The listing builds one solid part. Answer for the finished solid, in the listing's coordinates (mm). A direction names the side the tool comes from. Round coordinates to 2 decimals unless told otherwise and drop trailing zeros. Write each loop counter-clockwise with the first axis right and the second up, starting at its lowest first coordinate (ties: lowest second). Pieces come first, ordered by that corner, then holes. Notation, with made-up numbers: (-27.75, 51) - (25.25, 51) arc R17 ccw to (25.25, 71) - close; hole circle Ø1 at (-15, -36.75). An arc over 180 degrees is marked (long way). Return JSON: item names as keys, results as strings. Group by question number.
from build123d import *

# Parameters (mm, degrees)
SKETCH_1_W          = 107
SKETCH_1_H          = 94
EXTRUDE_1_DEPTH     = 8.5
SKETCH_2_W          = 104
SKETCH_2_H          = 91
CUT_EXTRUDE_1_DEPTH = 6.5
SKETCH_3_W          = 100
SKETCH_3_H          = 5.5
CUT_EXTRUDE_2_DEPTH = 6
SKETCH_4_W          = 10
SKETCH_4_H          = 15
EXTRUDE_2_DEPTH     = 2
FILLET_1_R          = 2
SKETCH_5_R          = 1.5
CUT_EXTRUDE_3_DEPTH = 3


with BuildPart() as part:
    # 草图1 → 凸台-拉伸1 (new body)
    with BuildSketch(Plane.XY):
        Rectangle(SKETCH_1_W, SKETCH_1_H)
    extrude(amount=EXTRUDE_1_DEPTH)

    # 草图2 → 切除-拉伸1 (cut)
    with BuildSketch(Plane(origin=(0, 0, 0), x_dir=(-1, 0, 0), z_dir=(0, 0, -1))):
        Rectangle(SKETCH_2_W, SKETCH_2_H)
    extrude(amount=-CUT_EXTRUDE_1_DEPTH, mode=Mode.SUBTRACT)

    # 草图3 → 切除-拉伸2 (cut)
    with BuildSketch(Plane.XZ.offset(47)):
        with Locations((0, 0.75)):
            Rectangle(SKETCH_3_W, SKETCH_3_H)
    extrude(amount=-CUT_EXTRUDE_2_DEPTH, mode=Mode.SUBTRACT)

    # 草图4 → 凸台-拉伸2 (add)
    with BuildSketch(Plane.XY.offset(8.5)):
        with Locations((58.5, 39.5)):
            Rectangle(SKETCH_4_W, SKETCH_4_H)
        with Locations((58.5, -39.5)):
            Rectangle(SKETCH_4_W, SKETCH_4_H)
        with Locations((-58.5, 39.5)):
            Rectangle(SKETCH_4_W, SKETCH_4_H)
        with Locations((-58.5, -39.5)):
            Rectangle(SKETCH_4_W, SKETCH_4_H)
    extrude(amount=-EXTRUDE_2_DEPTH)

    # 圆角1
    fillet_1_edges = [part.edges().sort_by_distance(p)[0] for p in [
        (63.5, 47, 7.5),
        (63.5, 32, 7.5),
        (63.5, -47, 7.5),
        (63.5, -32, 7.5),
        (-63.5, 47, 7.5),
        (-63.5, 32, 7.5),
        (-63.5, -47, 7.5),
        (-63.5, -32, 7.5),
    ]]
    fillet(fillet_1_edges, radius=FILLET_1_R)

    # 草图5 → 切除-拉伸3 (cut)
    with BuildSketch(Plane(origin=(0, 0, 6.5), x_dir=(-1, 0, 0), z_dir=(0, 0, -1))):
        with Locations((59, 39.5)):
            Circle(SKETCH_5_R)
        with Locations(Location((59, -39.5, 0), (0, 0, 180))):
            Circle(SKETCH_5_R)
        with Locations(Location((-59, 39.5, 0), (0, 0, 180))):
            Circle(SKETCH_5_R)
        with Locations((-59, -39.5)):
            Circle(SKETCH_5_R)
    extrude(amount=-CUT_EXTRUDE_3_DEPTH, mode=Mode.SUBTRACT)


solid = part.part
(1) Flat-ended cylindrical pins translate along their axes: pin 1 (2 mm diameter, centred on y = -0.5, z = 4.5, fed in from -X); pin 2 (11 mm diameter, centred on x = -60, y = 36.5, fed in from -Z); pin 3 (5 mm diameter, centred on y = -18.5, z = 5, fed in from +X). Find the tip coordinate at first contact, or state that the pin passes through.
(2) Determine the mould class of faces 4 (the flat face through (57, 40, 6.5)), 5 (the flat face through (52, -1, 3)), 6 (the flat face through (-1, -47, 6)) for opening direction Y: +Y half, -Y half, draft (parallel to the pull), parting line (faces both ways), or undercut.
(3) Consider line 1 (Y direction, x = 59, z = 7.25); line 2 (X direction, y = -40, z = 5.5); line 3 (Y direction, x = -20, z = 4.5). Determine where each line is inside the solid, lowest interval first.
(4) Find section C-C (x = 30). Write down the section's boundary in (y, z), plus the area to 3 significant figures.
(5) Find section B-B (y = 39.5). Write down the section's boundary in (x, z), plus the area to 4 significant figures.
(6) For faces 1 (the flat face through (-57, 40, 6.5)), 2 (the flat face through (1, -45.5, 5)), 3 (the flat face through (57, -39, 6.5)), determine the directions among +Z, -Z, +X, -X, +Y, -Y from which every point of the face is accessible in a straight line to the end or side of a thin tool.
(7) Find section D-D (y = 28.5). Write down the section's boundary in (x, z), plus the area to 4 significant figures.
(8) Find section A-A (x = 55.5). Write down the section's boundary in (y, z).
Check sheet entries:
{
 "1": {"pin 1": "stops at x = -53.5", "pin 2": "stops at z = 6.5", "pin 3": "stops at x = 53.5"},
 "2": {"face 4": "draft", "face 5": "undercut", "face 6": "-Y half"},
 "3": {"line 1": "y = -47 to -41, -38 to -32, 32 to 38, 41 to 47", "line 2": "x = -53.5 to -52, 52 to 53.5", "line 3": "y = -47 to -45.5, 45.5 to 47"},
 "4": {"outline": "(-47, 3.5) - (-45.5, 3.5) - (-45.5, 6.5) - (45.5, 6.5) - (45.5, 0) - (47, 0) - (47, 8.5) - (-47, 8.5) - close", "area": "202 mm^2"},
 "5": {"outline": "(-63.5, 6.5) - (-60.5, 6.5) - (-60.5, 8.5) - (-63.5, 8.5) - close; (-57.5, 6.5) - (-53.5, 6.5) - (-53.5, 0) - (-52, 0) - (-52, 6.5) - (52, 6.5) - (52, 0) - (53.5, 0) - (53.5, 6.5) - (57.5, 6.5) - (57.5, 8.5) - (-57.5, 8.5) - close; (60.5, 6.5) - (63.5, 6.5) - (63.5, 8.5) - (60.5, 8.5) - close", "area": "261.5 mm^2"},
 "6": {"face 1": "-Z, -X, +Y, -Y", "face 2": "-Z", "face 3": "-Z, +X, +Y, -Y"},
 "7": {"outline": "(-53.5, 0) - (-52, 0) - (-52, 6.5) - (52, 6.5) - (52, 0) - (53.5, 0) - (53.5, 8.5) - (-53.5, 8.5) - close", "area": "233.5 mm^2"},
 "8": {"outline": "(-47, 6.5) - (-32, 6.5) - (-32, 8.5) - (-47, 8.5) - close; (32, 6.5) - (47, 6.5) - (47, 8.5) - (32, 8.5) - close"}
}
